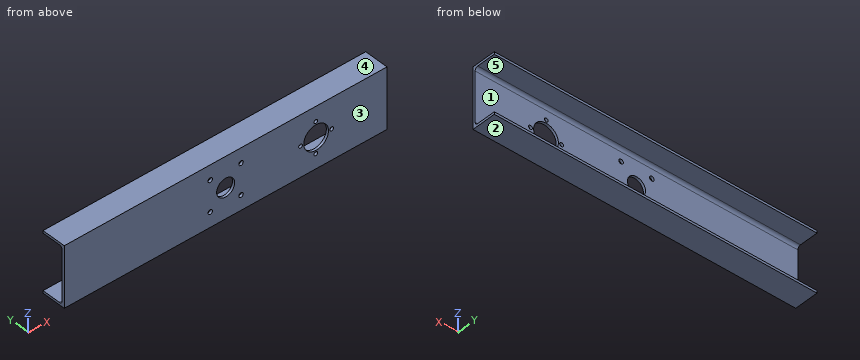
```python
from build123d import *

# Parameters (mm, degrees)
F0_W     = 1070
F0_H     = 200
F1_DEPTH = 80
F2_T     = -8
F3_D     = 60
F4_R     = 10
F5_D     = 15
F6_D     = 82
F7_D     = 12.5


with BuildPart() as f1:
    # F0 (on Front) → F1 (new body)
    with BuildSketch(Plane.XZ):
        Rectangle(F0_W, F0_H)
    extrude(amount=F1_DEPTH)

    # F2
    f2_openings = [f1.faces().sort_by_distance(p)[0] for p in [
        (0, 0, 0),
        (-535, -40, 0),
        (535, -40, 0),
    ]]
    offset(amount=F2_T, openings=f2_openings)

    # F3 (through all)
    with Locations(Plane(origin=(0, 0, 0), x_dir=(1, 0, 0), z_dir=(0, 1, 0))):
        with Locations((0, 0)):
            Hole(F3_D / 2)

    # F4
    f4_edges = [f1.edges().sort_by_distance(p)[0] for p in [
        (0, -72, -92),
        (0, -72, 92),
    ]]
    fillet(f4_edges, radius=F4_R)

    # F5 (through all)
    with Locations(Plane(origin=(0, 0, 0), x_dir=(1, 0, 0), z_dir=(0, 1, 0))):
        with Locations((-51, -51), (51, -51), (51, 51), (-51, 51)):
            Hole(F5_D / 2)

    # F6 (through all)
    with Locations(Plane(origin=(0, 0, 0), x_dir=(1, 0, 0), z_dir=(0, 1, 0))):
        with Locations((300, 0)):
            Hole(F6_D / 2)

    # F7 (through all)
    with Locations(Plane(origin=(0, 0, 0), x_dir=(1, 0, 0), z_dir=(0, 1, 0))):
        with Locations((248.5, 0.2018298983), (298.9653646946, -51.5), (351.5, 0.2018298983), (298.9653646946, 51.5)):
            Hole(F7_D / 2)


solid = f1.part
```
The model under review builds one solid part; all positions refer to its coordinate system, in mm. Face numbers are marked on the shaded views. A direction names the side the tool comes from. Give positions to 0.01 mm unless a question says otherwise; leave off trailing zeros. Write each loop counter-clockwise with the first axis right and the second up, starting at its lowest first coordinate (ties: lowest second). Pieces come first, ordered by that corner, then holes. Notation, with made-up numbers: M -34.5,-5.75 L 13.5,-5.75 A34 ccw 13.5,28.25 Z; hole C 43.5,78.5 d2. An arc over 180 degrees is marked long. Answer in a Markdown table with one row per item.
Item 1: Add section A-A on y = -26. Give the boundary of the cut face in (x, z).
Check sheet entries:
| item | result |
|---|---|
| outline | M -535,-100 L 535,-100 L 535,-92 L -535,-92 Z; M -535,92 L 535,92 L 535,100 L -535,100 Z |
Item 2: Tool access review of the marked faces 1 and 2: name each direction out of +Z, -Z, +X, -X, +Y, -Y from which nothing blocks a thin tool from reaching the whole face with its end or side.
Check sheet entries:
| item | result |
|---|---|
| face 1 | +X, -X, +Y |
| face 2 | -Z, +X, -X, +Y, -Y |
Item 3: Add section C-C on x = 207.5. Give the boundary of the cut face in (y, z).
Check sheet entries:
| item | result |
|---|---|
| outline | M -80,-100 L 0,-100 L 0,-92 L -62,-92 A10 cw -72,-82 L -72,82 A10 cw -62,92 L 0,92 L 0,100 L -80,100 Z |
Item 4: For line 1 along Z through (x, y) = (-51, -75.5); line 2 along X through (y, z) = (-77.5, 51); line 3 along Z through (x, y) = (-19.5, -33), list the stretches that pass through material, from the lowest coordinate up.
Check sheet entries:
| item | result |
|---|---|
| line 1 | -100 to -58.5, -43.5 to 43.5, 58.5 to 100 |
| line 2 | -535 to -58.5, -43.5 to 43.5, 58.5 to 292.74, 305.2 to 535 |
| line 3 | -100 to -92, 92 to 100 |
Item 5: Draft analysis for pull direction Z (two halves, no side actions). For the marked faces 3, 4 and 5, state which applies: +Z half, -Z half, draft (parallel to the pull), parting line (faces both ways), or undercut.
Check sheet entries:
| item | result |
|---|---|
| face 3 | draft |
| face 4 | +Z half |
| face 5 | undercut |
Item 6: Add section B-B on x = 0. Give the boundary of the cut face in (y, z), plus the area to 3 significant figures.
Check sheet entries:
| item | result |
|---|---|
| outline | M -80,-100 L 0,-100 L 0,-92 L -62,-92 A10 cw -72,-82 L -72,-30 L -80,-30 Z; M -80,30 L -72,30 L -72,82 A10 cw -62,92 L 0,92 L 0,100 L -80,100 Z |
| area | 2,310 mm2 |
Item 7: For P1, Ø16, axis at x = 298.97, z = 51.5, coming from the +Y side; P2, Ø19.5, axis at x = 51, z = -51, coming from the -Y side, all flat-tipped, find the tip position at first contact; note any pin that passes through.
Check sheet entries:
| item | result |
|---|---|
| P1 | y = -72 |
| P2 | y = -80 |
